```python
from build123d import *

# Parameters (mm, degrees)
BOSS_EXTRUDE1_DEPTH = 45.72
SKETCH3_R           = 2
CUT_EXTRUDE1_DEPTH  = 8
SKETCH4_R           = 1.27
CUT_EXTRUDE2_DEPTH  = 2.54


with BuildPart() as part:
    # Sketch1 → Boss-Extrude1 (new body)
    with BuildSketch(Plane.XY):
        Polygon((-132.98483419, 115.353503619), (-137.17583419, 108.094478684), (-128.79383419, 108.094478684), align=None)
    extrude(amount=BOSS_EXTRUDE1_DEPTH)

    # Sketch3 → Cut-Extrude1 (cut)
    with BuildSketch(Plane(origin=(0, 0, 0), x_dir=(-1, 0, 0), z_dir=(0, 0, -1))):
        with Locations((132.98483419, 110.514153662)):
            Circle(SKETCH3_R)
    extrude(amount=-CUT_EXTRUDE1_DEPTH, mode=Mode.SUBTRACT)

    # Sketch4 → Cut-Extrude2 (cut)
    with BuildSketch(Plane(origin=(-149.688157917, 86.422498268, 0), x_dir=(0, 0, 1), z_dir=(-0.8660254037844388, 0.4999999999999997, 0))):
        with Locations(Location((4, 29.215647454, 0), (0, 0, 270))):
            Circle(SKETCH4_R)
    extrude(amount=-CUT_EXTRUDE2_DEPTH, mode=Mode.SUBTRACT)


solid = part.part
```
Design review of the part built by this model. Coordinates are the model's own, in mm. A direction names the side the tool comes from. Round coordinates to 2 decimals unless told otherwise and drop trailing zeros. Write each loop counter-clockwise with the first axis right and the second up, starting at its lowest first coordinate (ties: lowest second). Pieces come first, ordered by that corner, then holes. Notation, with made-up numbers: (-16.5, 47) -> (28.5, 47) arc R37 cw to (28.5, 85) -> close; hole circle Ø10 at (89, 72.5). An arc over 180 degrees is marked (long way). Write item = value, one per line. Start each with the question number.
1) Mouldability with a two-part tool opening along Y and no side actions: class faces 3 (the face through (-135.1, 111, 5.1)), 4 (the face through (-133, 108.094, 23)), 5 (the face through (-135.051, 111.775, 22.54)), 6 (the face through (-134.9, 111.5, 0)) as +Y half, -Y half, draft (parallel to the pull), parting line (faces both ways), or undercut.
2) Wall thickness on probe 1 along Z at (x, y) = (-133.25, 111.75); probe 2 along X at (y, z) = (109, 2.5); probe 3 along X at (y, z) = (114.5, 43.5): over which ranges is each line inside the solid? List them lowest first. Write a range as from..to.
3) Clearance check with flat-ended pins moving along their axes: pin 1 (5 mm diameter, centred on x = -131.5, z = 37, fed in from +Y); pin 2 (1.2 mm diameter, centred on x = -133.5, y = 110, fed in from -Z); pin 3 (1.5 mm diameter, centred on x = -131.5, z = 35, fed in from +Y). State where each tip first meets the part, or that it passes through.
4) Take a section at C-C, the plane y = 113.25. State the section outline as (x, z) points.
5) Take a section at D-D, the plane x = -129.25. State the section outline as (y, z) points.
6) Take a section at B-B, the plane z = 34. State the section outline as (x, y) points.
7) Tool access review of faces 1 (the face through (-130.86, 111.67, 22.54)), 2 (the face through (-133, 111, 8)): name each direction out of +Z, -Z, +X, -X, +Y, -Y from which nothing blocks a thin tool from reaching the whole face with its end or side.
8) Take a section at A-A, the plane x = -132.5. State the section outline as (y, z) points.
Results list:
q1.face_3 = undercut
q1.face_4 = -Y half
q1.face_5 = +Y half
q1.face_6 = draft
q2.probe_1 = 8..45.72
q2.probe_2 = -136.65..-134.29, -131.68..-129.32
q2.probe_3 = -133.48..-132.49
q3.pin_1 = 115.35
q3.pin_2 = 8
q3.pin_3 = 114.08
q4.outline = (-134.2, 0) -> (-131.77, 0) -> (-131.77, 45.72) -> (-134.2, 45.72) -> close
q5.outline = (108.09, 0) -> (108.88, 0) -> (108.88, 45.72) -> (108.09, 45.72) -> close
q6.outline = (-137.18, 108.09) -> (-128.79, 108.09) -> (-132.98, 115.35) -> close
q7.face_1 = +Z, -Z, +X, +Y
q7.face_2 = -Z
q8.outline = (108.09, 0) -> (108.57, 0) -> (108.57, 8) -> (112.45, 8) -> (112.45, 0) -> (114.51, 0) -> (114.51, 45.72) -> (108.09, 45.72) -> close
